from build123d import *

# Parameters (mm, degrees)
SKETCH1_R           = 9.525
BOSS_EXTRUDE1_DEPTH = 10.16
FILLET1_R           = 16


with BuildPart() as part:
    # Sketch1 → Boss-Extrude1 (new body)
    with BuildSketch(Plane.XY):
        Polygon((0, 0), (0, 250), (195.1, 180), align=None)
        with Locations((165.1, 174.5)):
            Circle(SKETCH1_R, mode=Mode.SUBTRACT)
    extrude(amount=BOSS_EXTRUDE1_DEPTH)

    # Fillet1
    fillet1_edges = [part.edges().sort_by_distance(p)[0] for p in [
        (195.1, 180, 5.08),
    ]]
    fillet(fillet1_edges, radius=FILLET1_R)


solid = part.part
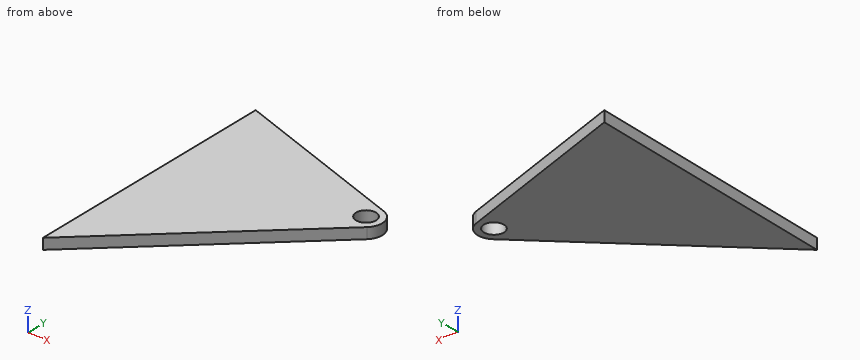
Source: CAD feature listing. Evaluate the final solid. Frame: model axes, mm. Coordinates: 2 decimals unless noted, no trailing zeros. Order: outer loops, then holes, each group sorted by start corner. A loop starts at its lowest first (then second) coordinate and runs counter-clockwise, first axis right, second up. Notation, with made-up numbers: M -32.75,20.5 L 9.25,20.5 A20 ccw 9.25,31.5 Z; hole C 25.5,88.5 d5. An arc over 180 degrees is marked long. Write each question's results on one line, items separated by ' | '. Start each with the question number.
Item 1: Line query: probe 1 along Y at (x, z) = (165.1, 3) (3 decimals); probe 2 along Y at (x, z) = (157.5, 6.25); probe 3 along X at (y, z) = (182, 3.5). Output: solid intervals per line, ascending.
Item 2: First-contact query: pin 1 Ø15 at (x, y) = (165.1, 174.5) entering from +Z; pin 2 Ø1.5 at (x, z) = (64, 7.5) entering from -Y; pin 3 Ø1.5 at (y, z) = (48, 2.5) entering from +X; pin 4 Ø12 at (x, y) = (92, 153.5) entering from -Z. Flat tips, straight axial feed; report the tip coordinate or a pass-through.
Item 3: Cut plane D-D (x = 32). Return loops of the section in (y, z), and give its area (3 significant figures).
Item 4: Cut plane C-C (y = 170.5). Return loops of the section in (x, z), and give its area (3 significant figures).
Item 5: Cut plane A-A (z = 5.5). Return loops of the section in (x, y) (3 decimals).
Item 6: Cut plane B-B (x = 165.1). Return loops of the section in (y, z) (3 decimals).
Checked values:
1) probe 1: y = 152.322 to 164.975, 184.025 to 190.764 | probe 2: y = 145.31 to 168.76, 180.24 to 193.49 | probe 3: x = 0 to 159.23, 170.97 to 178.62
2) pin 1: passes through | pin 2: stops at y = 58.35 | pin 3: stops at x = 52.84 | pin 4: stops at z = 0
3) outline: M 29.52,0 L 238.52,0 L 238.52,10.16 L 29.52,10.16 Z | area: 2,120 mm2
4) outline: M 0,0 L 156.46,0 L 156.46,10.16 L 0,10.16 Z; M 173.74,0 L 180.49,0 L 180.49,10.16 L 173.74,10.16 Z | area: 1,660 mm2
5) outline: M 0,0 L 175.695,162.097 A16 ccw 170.249,188.916 L 0,250 Z; hole C 165.1,174.5 d19.05
6) outline: M 152.322,0 L 164.975,0 L 164.975,10.16 L 152.322,10.16 Z; M 184.025,0 L 190.764,0 L 190.764,10.16 L 184.025,10.16 Z
